Here's the drawing with two shaded views (mm, measured from the low corner). I have some questions. Give positions to 0.01 mm unless a question says otherwise; leave off trailing zeros. Loops run counter-clockwise (first coordinate to the right, second up) from the corner with the lowest first, then second, coordinate; pieces in that order, holes last. Notation, with made-up numbers: M 73,-21 L 91,-21 A22 ccw 91,2 Z; hole C 77,-20 d11. An arc over 180 degrees is marked long. Put each result on its own line as item: value. Start each with the question number.
1) Imagine slicing it at C-C (x = 91). Write out the boundary of the cut face in (y, z).
2) Imagine slicing it at A-A (z = 27.5). Write out the boundary of the cut face in (x, y).
3) For P1, Ø1.5, axis at x = 46.5, z = 33, coming from the +Y side, with a flat end and sliding along its axis, tell me the tip position at first contact or that it passes through.
4) Please list where these lines run through material, in increasing order: line 1 along Z through (x, y) = (17, 7); line 2 along X through (y, z) = (7.5, 52); line 3 along Y through (x, z) = (38, 86.5). Write a range as from..to.
5) Imagine slicing it at B-B (y = 6.5). Write out the boundary of the cut face in (x, z).
6) If we mould it in two halves opening along Z, with no side actions, what happens to the marked faces 1 and 2? For each: +Z half, -Z half, draft (parallel to the pull), parting line (faces both ways), or undercut.
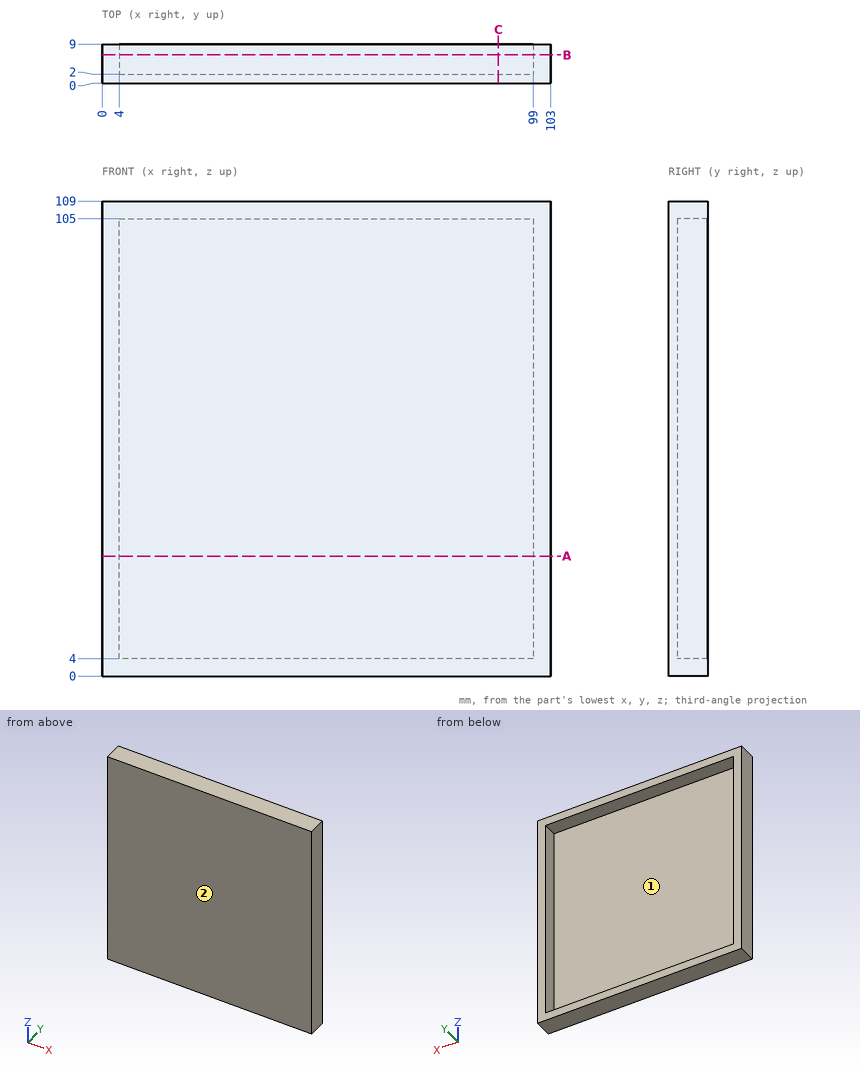
Recorded:
1. outline: M 0,0 L 9,0 L 9,4 L 2,4 L 2,105 L 9,105 L 9,109 L 0,109 Z
2. outline: M 0,0 L 103,0 L 103,9 L 99,9 L 99,2 L 4,2 L 4,9 L 0,9 Z
3. P1: y = 2
4. line 1: 0..4, 105..109
4. line 2: 0..4, 99..103
4. line 3: 0..2
5. outline: M 0,0 L 103,0 L 103,109 L 0,109 Z; hole M 4,4 L 99,4 L 99,105 L 4,105 Z
6. face 1: undercut
6. face 2: draft
